Verification items for the finished model (mm, model axes). A direction names the side the tool comes from. Round coordinates to 2 decimals unless told otherwise and drop trailing zeros. Write each loop counter-clockwise with the first axis right and the second up, starting at its lowest first coordinate (ties: lowest second). Pieces come first, ordered by that corner, then holes. Notation, with made-up numbers: M 34.25,42 L 74.25,42 A23 ccw 74.25,68 Z; hole C 64.25,-8 d6. An arc over 180 degrees is marked long. Use a Markdown table: item, result. Add a question column.
Autodesk Inventor part; units mm, degrees
ref_plane "YZ Plane" through (0, 0, 0) normal (1, 0, 0) x (0, 1, 0)
ref_plane "XZ Plane" through (0, 0, 0) normal (0, 1, 0) x (-1, 0, 0)
ref_plane "XY Plane" through (0, 0, 0) normal (0, 0, 1) x (1, 0, 0)
sketch "Skizze3" plane through (0, 0, 0) normal (1, 0, 0) x (0, 1, 0)
  line L0 (4.8, 5) -> (-4.8, 5)
  line L1 (2.9, 5) -> (2.9, 25)
  line L2 (2.9, 25) -> (-2.9, 25)
  line L3 (-2.9, 25) -> (-2.9, 5)
  line L4 (-2.9, 25) -> (-4.8, 25)
  line L5 (-4.8, 25) -> (-4.8, 7)
  line L6 (-4.8, 7) -> (-2.9, 7)
  line L7 (2.9, 7) -> (4.8, 7)
  line L8 (4.8, 7) -> (4.8, 25)
  line L9 (4.8, 25) -> (2.9, 25)
  line L10 (0, -5) -> (0, 30)
  line L11 (4.8, 5) -> (4.8, 2.5)
  line L12 (-2.9, 0) -> (-4.8, 2.5)
  line L13 (-4.8, 2.5) -> (-4.8, 5)
  line L14 (4.8, 2.5) -> (2.9, 0)
  line L15 (2.9, 0) -> (-2.9, 0)
  line L16 (-6.72, 0) -> (6.72, 0)
  line L17 (-2.9, 0) -> (-4.8, 0)
  line L18 (-4.8, 2.5) -> (-4.8, 0)
  line L19 (4.8, 2.5) -> (4.8, 0)
  line L20 (4.8, 0) -> (2.9, 0)
  line L21 (4.8, 5) -> (4.8, 7)
  line L22 (-4.8, 5) -> (-4.8, 7)
  point P0 (0, 0)
  point P1 (0, 25)
  point P2 (0, 5)
  point P3 (0, 0)
  point P4 (0, 16)
  dimension "d5" = 9.6
  dimension "d6" = 5.8
  dimension "d7" = 1.9
  dimension "d9" = 18
  dimension "d10" = 18
  dimension "d12" = 9.6
  dimension "d14" = 2.9
  dimension "d15" = 2.5
  dimension "d16" = 5.8
  dimension "d17" = 2.5
  dimension "d18" = 5
  dimension "d19" = 25
  dimension "d40" = 9
sketch "Skizze4" plane through (0, 0, 0) normal (0, 1, 0) x (-1, 0, 0)
  line L0 (0, 25) -> (0, 7)
  line L1 (0, 2.5) -> (0, 5)
  line L2 (0, 0) -> (0, 25)
  line L3 (0, 25) -> (-5.8, 25)
  line L4 (-5.8, 25) -> (-5.8, 5.8)
  line L5 (-5.8, 5.8) -> (-26, 5.8)
  line L6 (-26, 5.8) -> (-26, 0)
  line L7 (-26, 0) -> (0, 0)
  line L8 (-0.65, 25) -> (-0.65, 7)
  line L9 (-0.65, 7) -> (-5.15, 7)
  line L10 (-5.15, 7) -> (-5.15, 25)
  line L11 (-1, 0) -> (-1, 5)
  line L12 (-1, 5) -> (-26, 5)
  line L13 (-1, 0) -> (-5, 2.5)
  line L14 (-5, 2.5) -> (-22, 2.5)
  line L15 (-22, 2.5) -> (-26, 0)
  line L16 (-22, 2.5) -> (-22, 5)
  line L17 (-5, 2.5) -> (-5, 5)
  point P0 (0, 0)
  point P1 (0, 0)
  dimension "d20" = 5.8
  dimension "d21" = 4.5
  dimension "d22" = 0.65
  dimension "d23" = 26
  dimension "d24" = 5.8
  dimension "d25" = 25
  dimension "d26" = 4
  dimension "d27" = 4
sketch "Skizze5" plane through (0, 0, 0) normal (0, 0, 1) x (1, 0, 0)
  line L0 (5.15, 4.8) -> (0.65, 4.8)
  line L1 (0.65, 4.8) -> (0.65, 2.9)
  line L2 (0.65, 2.9) -> (0, 2.9)
  line L3 (0, 2.9) -> (0, -2.9)
  line L4 (0, -2.9) -> (0.65, -2.9)
  line L5 (0.65, -2.9) -> (0.65, -4.8)
  line L6 (0.65, -4.8) -> (5.15, -4.8)
  line L7 (5.15, -4.8) -> (5.15, -2.9)
  line L8 (5.15, -2.9) -> (5.8, -2.9)
  line L9 (5.8, -2.9) -> (5.8, 2.9)
  line L10 (5.8, 2.9) -> (5.15, 2.9)
  line L11 (5.15, 4.8) -> (5.15, 2.9)
  line L12 (0, -2.9) -> (26, -2.9)
  line L13 (26, -2.9) -> (26, 2.9)
  line L14 (26, 2.9) -> (0, 2.9)
  line L15 (26, -2.9) -> (22, -4.8)
  line L16 (22, -4.8) -> (5, -4.8)
  line L17 (1, -2.9) -> (5, -4.8)
  line L18 (22, -7.8717) -> (22, 8.228) construction
  line L19 (5, -6.3703) -> (5, 8.228) construction
  line L20 (1, -9.3021) -> (1, 6.7781) construction
  line L21 (26, 2.9) -> (22, 4.8)
  line L22 (5, 4.8) -> (1, 2.9)
  line L23 (5, 4.8) -> (22, 4.8)
  line L24 (26, 0) -> (0, 0)
  point P0 (5.8, 0)
  point P1 (5.15, 0)
  point P2 (0.65, 0)
  point P3 (0, 4.8)
  point P4 (0, -4.8)
  point P5 (1, 0)
  point P6 (1, 0)
  point P7 (1, 0)
  point P8 (5, 0)
  point P9 (5, 0)
  point P10 (5, 0)
  point P11 (22, 0)
  point P12 (22, 0)
  point P13 (22, 0)
  point P14 (26, 0)
  point P15 (26, 0)
  point P16 (20, 0)
  dimension "d41" = 6
extrude "Extrusion6" add sketch "Skizze5" along normal blind 25 contours L11 L14 L22 L0 | L22 L14 L1 L0 | L10 L9 L24 L3 L2 L14 | L9 L8 L12 L4 L3 L24 | L7 L6 L17 L12 | L17 L6 L5 L12
extrude "Extrusion7" cut sketch "Skizze3" along normal through all contours L0 L1 L7 L21 | L0 L22 L6 L3
extrude "Extrusion3" add sketch "Skizze5" along normal blind 5 separate body contours L11 L14 L22 L0 | L23 L21 L14 L10 L11 | L10 L9 L24 L3 L2 L14 | L14 L13 L24 L9 | L24 L13 L12 L9 | L9 L8 L12 L4 L3 L24 | L12 L15 L16 L7 L8 | L7 L6 L17 L12
extrude "Extrusion5" add sketch "Skizze5" along normal blind 5.8 contours L14 L13 L24 L9 | L24 L13 L12 L9
extrude "Extrusion4" cut sketch "Skizze3" along normal through all contours L19 L16 L14 | L16 L18 L12
extrude "Extrusion8" cut sketch "Skizze5" along normal up to surface (5 mm away) contours L22 L14 L1 L0 | L17 L6 L5 L12
hole "Bohrung1" at (20, 0, 0) direction (0, 0, 1) diameter 3.242 end through all
hole "Bohrung2" at (0, 0, 16) direction (1, 0, 0) diameter 3.242 end through all
chamfer "Fase1" distance 0.2 angle 45 4 edges at (0, 0, 14.379) (5.8, 0, 14.379) (20, -1.621, 5.8) (20, -1.621, 0)
equation "\"d5\" = H2"
equation "\"d6\" = H1"
equation "\"d7\" = -0.5 * d6 + 0.5 * d5"
equation "\"d12\" = d5"
equation "\"d14\" = 0.5 * d16"
equation "\"d19\" = L2"
equation "\"d20\" = G2"
equation "\"d21\" = G1"
equation "\"d22\" = -0.5 * d21 + 0.5 * d20"
equation "\"d23\" = L1"
equation "\"d24\" = G2"
equation "\"d34\" = L2"
equation "\"d32\" = d24"
equation "\"d38\" = L2"
equation "\"L1\" = 26"
equation "\"L2\" = 25"
equation "\"H1\" = 5.8"
equation "\"H2\" = 9.6"
equation "\"G1\" = 4.5"
equation "\"G2\" = 5.8"
equation "\"M\" = 4"
properties part number "BT000_trajan20_21"
1. Cross-section at A-A on x = 20. Enter the section's corners in (y, z).
2. Cross-section at B-B on y = 0. Enter the section's corners in (x, z).
3. Depth check by flat-ended pin: pin 1 Ø3 at (y, z) = (-1, 18.5) entering from +X; pin 2 Ø1.9 at (y, z) = (0, 16) entering from -X; pin 3 Ø2 at (y, z) = (4, 15.5) entering from +X; pin 4 Ø2 at (x, y) = (3.5, 4) entering from -Z. Enter the tip coordinate at first touch or a pass-through.
4. Cross-section at C-C on z = 1.5. Enter the section's corners in (x, y), plus the area to 3 significant figures.
5. Cross-section at D-D on z = 16. Enter the section's corners in (x, y), plus the area to 3 significant figures.
6. Access from +Z, -Z, +X, -X, +Y, -Y to the whole of each face (thin tool, end or side, straight path). Record for faces 5 (the flat face through (3, -4, 7)), 6 (the flat face through (2.972, -3.837, 3.021)), 7 (the flat face through (5.15, 4, 16)), 8 (the flat face through (3.028, 3.863, 3.021)).
7. Scan lines: line 1 along X through (y, z) = (0, 3.4); line 2 along Y through (x, z) = (20, 3.3); line 3 along Z through (x, y) = (3.5, 0). Record each from-to range of solid material in increasing order. Write a range as from..to.
8. Release check for a two-part mould opening along Y. For faces 1 (the flat face through (13.325, -3.837, 1.232)), 2 (the cylindrical face through (21.582, -0.351, 2.938)), 3 (the flat face through (5.15, -4, 16)), 4 (the flat face through (14, 4.8, 4)) record: +Y half, -Y half, draft (parallel to the pull), parting line (faces both ways), or undercut.
Answer:
| question | item | result |
|---|---|---|
| 1 | outline | M -4.8,2.5 L -2.9,0 L -1.82,0 L -1.62,0.2 L -1.62,5.6 L -1.82,5.8 L -2.9,5.8 L -2.9,5 L -4.8,5 Z; M 1.62,0.2 L 1.82,0 L 2.9,0 L 4.8,2.5 L 4.8,5 L 2.9,5 L 2.9,5.8 L 1.82,5.8 L 1.62,5.6 Z |
| 2 | outline | M 0,0 L 18.18,0 L 18.38,0.2 L 18.38,5.6 L 18.18,5.8 L 5.8,5.8 L 5.8,14.18 L 5.6,14.38 L 0.2,14.38 L 0,14.18 Z; M 0,17.82 L 0.2,17.62 L 5.6,17.62 L 5.8,17.82 L 5.8,25 L 0,25 Z; M 21.62,0.2 L 21.82,0 L 26,0 L 26,5.8 L 21.82,5.8 L 21.62,5.6 Z |
| 3 | pin 1 | stops at x = 5.8 |
| 3 | pin 2 | passes through |
| 3 | pin 3 | stops at x = 5.15 |
| 3 | pin 4 | stops at z = 0.13 |
| 4 | outline | M 0,-2.9 L 1,-2.9 L 3.4,-4.04 L 23.6,-4.04 L 26,-2.9 L 26,2.9 L 23.6,4.04 L 3.4,4.04 L 1,2.9 L 0,2.9 Z; hole C 20,0 d3.24 |
| 4 | area | 194 mm^2 |
| 5 | outline | M 0,-2.9 L 0.65,-2.9 L 0.65,-4.8 L 5.15,-4.8 L 5.15,-2.9 L 5.8,-2.9 L 5.8,-1.82 L 5.6,-1.62 L 0.2,-1.62 L 0,-1.82 Z; M 0,1.82 L 0.2,1.62 L 5.6,1.62 L 5.8,1.82 L 5.8,2.9 L 5.15,2.9 L 5.15,4.8 L 0.65,4.8 L 0.65,2.9 L 0,2.9 Z |
| 5 | area | 31.9 mm^2 |
| 6 | face 5 | +X, -X, -Y |
| 6 | face 6 | -Z, -X, -Y |
| 6 | face 7 | +Z, +X, +Y |
| 6 | face 8 | -Z, -X, +Y |
| 7 | line 1 | x = 0..18.38, 21.62..26 |
| 7 | line 2 | y = -4.8..-1.62, 1.62..4.8 |
| 7 | line 3 | z = 0..14.38, 17.62..25 |
| 8 | face 1 | -Y half |
| 8 | face 2 | undercut |
| 8 | face 3 | draft |
| 8 | face 4 | +Y half |
